Autodesk Inventor part; units mm, degrees
ref_plane "工作平面1" through (0, 0, 25) normal (0, 0, 1) x (1, 0, 0)
ref_plane "YZ Plane" through (0, 0, 0) normal (1, 0, 0) x (0, 1, 0)
ref_plane "XZ Plane" through (0, 0, 0) normal (0, 1, 0) x (-1, 0, 0)
sketch "草图1" plane through (0, 0, 0) normal (0, 0, 1) x (1, 0, 0)
  line L0 (-10, 0) -> (10, 0)
  line L1 (10, 0) -> (10, 29)
  line L2 (10, 29) -> (8, 29)
  line L3 (8, 29) -> (5.6906, 25)
  line L4 (5.6906, 25) -> (-5.6906, 25)
  line L5 (-5.6906, 25) -> (-8, 29)
  line L6 (-8, 29) -> (-10, 29)
  line L7 (-10, 29) -> (-10, 0)
  line L8 (-14, 0) -> (14, 0)
  point P0 (0, 0)
  point P1 (0, 0)
  dimension "d1" = 29
  dimension "d2" = 4
  dimension "d4" = 20
  dimension "d5" = 2
  dimension "d6" = 120
  dimension "d7" = 120
  dimension "d8" = 2
revolve "旋转1" add sketch "草图1" angle 360 about axis through (-10, 0, 0) along (1, 0, 0)
sketch "草图2" plane through (10, 0, 0) normal (1, 0, 0) x (0, 0, -1)
  circle A0 centre (0, 0) radius 10
  dimension "d10" = 20
extrude "拉伸1" cut sketch "草图2" against normal through all
ref_plane "工作平面1" through (0, 0, 25) normal (0, 0, 1) x (1, 0, 0)
sketch "草图3" plane through (0, 0, 25) normal (0, 0, 1) x (1, 0, 0)
  circle A0 centre (0, 0) radius 2
  dimension "d13" = 4
extrude "拉伸2" cut sketch "草图3" against normal up to surface
thread "螺纹1"
properties part number "砂轮电机皮带轮"
Geometry: final body of the model. Coordinates: model frame, mm. A direction names the side the tool comes from. Round coordinates to 2 decimals unless told otherwise and drop trailing zeros. Loops run counter-clockwise (first coordinate to the right, second up) from the corner with the lowest first, then second, coordinate; pieces in that order, holes last. Notation, with made-up numbers: M -34,45.5 L 15,45.5 A28 cw 15,80.5 Z; hole C -7.5,3.25 d2. An arc over 180 degrees is marked long. Put each result on its own line as item: value. Start each with the question number.
(1) Set-up query: faces 4 (the face through (-10, 12, 0)), 5 (the face through (-5.835, -25.226, -1.11)), 6 (the face through (0, -2, 18)). Return all of +Z, -Z, +X, -X, +Y, -Y with unobstructed straight access to the full face (end or side cutting, diameter ignored); none if empty.
(2) Section query A-A (y = 0). Return loops of the section in (x, z), then the cut area to 3 significant figures.
(3) Draft query along Y for faces 1 (the face through (10, 12, 0)), 2 (the face through (5.835, 11.651, -22.401)), 3 (the face through (0.14, 3, -9.54)). Return one class per face: +Y half, -Y half, draft (parallel to the pull), parting line (faces both ways), or undercut.
(4) Section query D-D (x = 0). Return loops of the section in (y, z), then the cut area to 3 significant figures.
(5) Section query B-B (z = 0). Return loops of the section in (x, y).
(6) Section query C-C (x = -4.75). Return loops of the section in (y, z), then the cut area to 3 significant figures.
(7) Material intervals for line 1 along Z through (x, y) = (5.5, 0); line 2 along X through (y, z) = (0, 14.25); line 3 along X through (y, z) = (-25, 9), sorted ascending. Write a range as [from, to].
(8) Contact query for flat-ended pins moving along their axis: pin 1 Ø2 at (x, y) = (6, -1) entering from -Z; pin 2 Ø8 at (x, z) = (1, -20) entering from -Y; pin 3 Ø3 at (x, y) = (-4, -15.5) entering from +Z; pin 4 Ø18 at (y, z) = (0, 0) entering from -X. Output: stop coordinate, or through.
Findings below:
1. face 4: +Z, -Z, -X, +Y, -Y
1. face 5: none
1. face 6: +Z
2. outline: M -10,-29 L -8,-29 L -5.69,-25 L 5.69,-25 L 8,-29 L 10,-29 L 10,-10 L -10,-10 Z; M -10,10 L -2,10 L -2,25 L -5.69,25 L -8,29 L -10,29 Z; M 2,10 L 10,10 L 10,29 L 8,29 L 5.69,25 L 2,25 Z
2. area: 590 mm2
3. face 1: draft
3. face 2: parting line
3. face 3: undercut
4. outline: M -2,9.8 L -2,24.92 A25 ccw long 2,24.92 L 2,9.8 A10 cw long Z
4. area: 1,590 mm2
5. outline: M -10,-29 L -8,-29 L -5.69,-25 L 5.69,-25 L 8,-29 L 10,-29 L 10,-10 L -10,-10 Z; M -10,10 L 10,10 L 10,29 L 8,29 L 5.69,25 L -5.69,25 L -8,29 L -10,29 Z
6. outline: C 0,0 d50; hole C 0,0 d20
6. area: 1,650 mm2
7. line 1: z = [-25, -10], [10, 25]
7. line 2: x = [-10, -2], [2, 10]
7. line 3: x = [-10, -6.6], [6.6, 10]
8. pin 1: stops at z = -27.25
8. pin 2: stops at y = -19.21
8. pin 3: stops at z = 20.71
8. pin 4: passes through
